For this review, take the finished solid that the model builds, in its own axes (mm). Face numbers are marked on the shaded views. A direction names the side the tool comes from. Round coordinates to 2 decimals unless told otherwise and drop trailing zeros. Loops run counter-clockwise (first coordinate to the right, second up) from the corner with the lowest first, then second, coordinate; pieces in that order, holes last. Notation, with made-up numbers: (3.25, 12.5) -> (34.25, 12.5) arc R14 ccw to (34.25, 21.5) -> close; hole circle Ø8 at (29, 75.5). An arc over 180 degrees is marked (long way). Write each question's results on one line, items separated by ' | '.
```python
from build123d import *

# Parameters (mm, degrees)
BOSS_EXTRUDE1_DEPTH = 5
SKETCH2_W           = 9
SKETCH2_H           = 5
SKETCH2_W_2         = 18
BOSS_EXTRUDE2_DEPTH = 9
SKETCH3_W           = 1.5
SKETCH3_H           = 9
SKETCH3_W_2         = 3.027864045
SKETCH3_W_3         = 2
SKETCH3_W_4         = 5.05572809
CUT_EXTRUDE1_DEPTH  = 228
BOSS_EXTRUDE3_DEPTH = 20
SKETCH5_W           = 11.583853266
SKETCH5_H           = 8
CUT_EXTRUDE3_DEPTH  = 20
SKETCH6_R           = 1.5
CUT_EXTRUDE5_DEPTH  = 25


with BuildPart() as part:
    # Sketch1 → Boss-Extrude1 (new body)
    with BuildSketch(Plane(origin=(0, 0, 0), x_dir=(1, 0, 0), z_dir=(0, 1, 0))):
        with BuildLine():
            Line((-64, 250), (-64, 0))
            ThreePointArc((-64, 0), (0, -64), (64, 0))
            Line((64, 0), (64, 250))
            ThreePointArc((64, 250), (0, 314), (-64, 250))
        make_face()
    extrude(amount=BOSS_EXTRUDE1_DEPTH)

    # Sketch2 → Boss-Extrude2 (add)
    with BuildSketch(Plane(origin=(0, 5, 0), x_dir=(1, 0, 0), z_dir=(0, 1, 0))):
        with Locations((4.5, 27.5)):
            Rectangle(SKETCH2_W, SKETCH2_H)
        with Locations((-4.5, 27.5)):
            Rectangle(SKETCH2_W, SKETCH2_H)
        with Locations((-53.5, 27.5)):
            Rectangle(SKETCH2_W, SKETCH2_H)
        with Locations((53.5, 27.5)):
            Rectangle(SKETCH2_W, SKETCH2_H)
        with Locations((53.5, 82.5)):
            Rectangle(SKETCH2_W, SKETCH2_H)
        with Locations((4.5, 82.5)):
            Rectangle(SKETCH2_W, SKETCH2_H)
        with Locations((-4.5, 82.5)):
            Rectangle(SKETCH2_W, SKETCH2_H)
        with Locations((-53.5, 82.5)):
            Rectangle(SKETCH2_W, SKETCH2_H)
        with Locations((-53.5, 137.5)):
            Rectangle(SKETCH2_W, SKETCH2_H)
        with Locations((-4.5, 137.5)):
            Rectangle(SKETCH2_W, SKETCH2_H)
        with Locations((4.5, 137.5)):
            Rectangle(SKETCH2_W, SKETCH2_H)
        with Locations((53.5, 137.5)):
            Rectangle(SKETCH2_W, SKETCH2_H)
        with Locations((53.5, 192.5)):
            Rectangle(SKETCH2_W, SKETCH2_H)
        with Locations((-53.5, 192.5)):
            Rectangle(SKETCH2_W, SKETCH2_H)
        with Locations((-53.5, 247.5)):
            Rectangle(SKETCH2_W, SKETCH2_H)
        with Locations((-4.5, 247.5)):
            Rectangle(SKETCH2_W, SKETCH2_H)
        with Locations((4.5, 247.5)):
            Rectangle(SKETCH2_W, SKETCH2_H)
        with Locations((53.5, 247.5)):
            Rectangle(SKETCH2_W, SKETCH2_H)
        with Locations((0, 192.5)):
            Rectangle(SKETCH2_W_2, SKETCH2_H)
    extrude(amount=BOSS_EXTRUDE2_DEPTH)

    # Sketch3 → Cut-Extrude1 (cut)
    with BuildSketch(Plane.XY.offset(-25)):
        with BuildLine():
            ThreePointArc((-56.5, 14), (-54.263932023, 12), (-52.027864045, 14))
            Line((-52.027864045, 14), (-56.5, 14))
        make_face()
        with Locations((-57.25, 9.5)):
            Rectangle(SKETCH3_W, SKETCH3_H)
        with Locations((-50.513932023, 9.5)):
            Rectangle(SKETCH3_W_2, SKETCH3_H)
        with Locations((-8, 9.5)):
            Rectangle(SKETCH3_W_3, SKETCH3_H)
        with BuildLine():
            Line((-2.527864045, 14), (-7, 14))
            ThreePointArc((-7, 14), (-4.763932023, 12), (-2.527864045, 14))
        make_face()
        with Locations((0, 9.5)):
            Rectangle(SKETCH3_W_4, SKETCH3_H)
        with BuildLine():
            Line((7, 14), (2.527864045, 14))
            ThreePointArc((2.527864045, 14), (4.763932023, 12), (7, 14))
        make_face()
        with Locations((8, 9.5)):
            Rectangle(SKETCH3_W_3, SKETCH3_H)
        with Locations((50.513932023, 9.5)):
            Rectangle(SKETCH3_W_2, SKETCH3_H)
        with BuildLine():
            Line((56.5, 14), (52.027864045, 14))
            ThreePointArc((52.027864045, 14), (54.263932023, 12), (56.5, 14))
        make_face()
        with Locations((57.25, 9.5)):
            Rectangle(SKETCH3_W, SKETCH3_H)
    extrude(amount=-CUT_EXTRUDE1_DEPTH, mode=Mode.SUBTRACT)

    # Sketch4 → Boss-Extrude3 (add)
    with BuildSketch(Plane.XZ):
        with BuildLine():
            Line((-64, 0), (-64, -250))
            ThreePointArc((-64, -250), (0, -314), (64, -250))
            Line((64, -250), (64, 0))
            ThreePointArc((64, 0), (0, 64), (-64, 0))
        make_face()
        with BuildLine():
            Line((-59, 0), (-59, -250))
            ThreePointArc((-59, -250), (0, -309), (59, -250))
            Line((59, -250), (59, 0))
            ThreePointArc((59, 0), (0, 59), (-59, 0))
        make_face(mode=Mode.SUBTRACT)
    extrude(amount=BOSS_EXTRUDE3_DEPTH)

    # Sketch5 → Cut-Extrude3 (cut)
    with BuildSketch(Plane(origin=(0, 5, 0), x_dir=(1, 0, 0), z_dir=(0, 1, 0))):
        with Locations((-50.708073367, 254)):
            Rectangle(SKETCH5_W, SKETCH5_H)
        with Locations((-50.708073367, 199)):
            Rectangle(SKETCH5_W, SKETCH5_H)
        with Locations((-50.708073367, 144)):
            Rectangle(SKETCH5_W, SKETCH5_H)
        with Locations((-50.708073367, 89)):
            Rectangle(SKETCH5_W, SKETCH5_H)
        with Locations((-50.708073367, 34)):
            Rectangle(SKETCH5_W, SKETCH5_H)
        with Locations((50.708073367, 144)):
            Rectangle(SKETCH5_W, SKETCH5_H)
        with Locations((50.708073367, 199)):
            Rectangle(SKETCH5_W, SKETCH5_H)
        with Locations((50.708073367, 254)):
            Rectangle(SKETCH5_W, SKETCH5_H)
        with Locations((50.708073367, 89)):
            Rectangle(SKETCH5_W, SKETCH5_H)
        with Locations((50.708073367, 34)):
            Rectangle(SKETCH5_W, SKETCH5_H)
    extrude(amount=-CUT_EXTRUDE3_DEPTH, mode=Mode.SUBTRACT)

    # Sketch6 → Cut-Extrude5 (cut)
    with BuildSketch(Plane.XZ):
        with Locations(Location((0, 54.47166112, 0), (0, 0, 270))):
            Circle(SKETCH6_R)
        with Locations(Location((0, -304.513619398, 0), (0, 0, 270))):
            Circle(SKETCH6_R)
    extrude(amount=-CUT_EXTRUDE5_DEPTH, mode=Mode.SUBTRACT)


solid = part.part
```
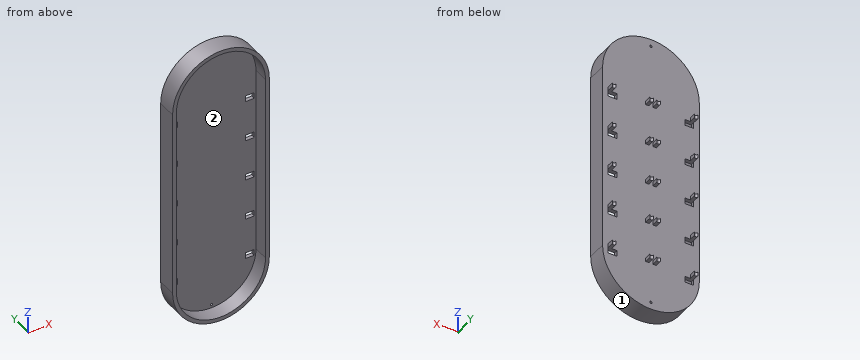
1. For pin 1 (5 mm diameter, centred on x = -5, y = 9.5, fed in from +Z); pin 2 (5.5 mm diameter, centred on y = 8.5, z = -26.5, fed in from +X); pin 3 (1.5 mm diameter, centred on y = 8.5, z = -136.5, fed in from -X), all flat-tipped, find the tip position at first contact; note any pin that passes through.
Values found:
pin 1: stops at z = -25 | pin 2: stops at x = 56.5 | pin 3: stops at x = -56.5
2. Consider section C-C (x = 29). State the section outline as (y, z) points.
Values found:
outline: (-20, -307.05) -> (5, -307.05) -> (5, 57.05) -> (-20, 57.05) -> (-20, 51.38) -> (0, 51.38) -> (0, -301.38) -> (-20, -301.38) -> close
3. Consider section B-B (z = -21.5). State the section outline as (x, y) points.
Values found:
outline: (-64, -20) -> (-59, -20) -> (-59, 0) -> (59, 0) -> (59, -20) -> (64, -20) -> (64, 5) -> (-64, 5) -> close
4. To check wall thickness, follow probe 1 along X at (y, z) = (-15, -12.5); probe 2 along Y at (x, z) = (49, -23); probe 3 along Z at (x, y) = (-52, 1). State the ranges of each line that lie inside material, in increasing order.
Values found:
probe 1: x = -64 to -59, 59 to 64 | probe 2: y = 0 to 5 | probe 3: z = -287.31 to -258, -250 to -203, -195 to -148, -140 to -93, -85 to -38, -30 to 37.31
5. Tool access review of the marked faces 1 and 2: name each direction out of +Z, -Z, +X, -X, +Y, -Y from which nothing blocks a thin tool from reaching the whole face with its end or side.
Values found:
face 1: -Z, +Y, -Y | face 2: -Y
6. Consider section A-A (y = -14.5). State the section outline as (x, z) points, plus the area to 3 significant figures.
Values found:
outline: (-64, -250) arc R64 ccw to (64, -250) -> (64, 0) arc R64 ccw to (-64, 0) -> close; hole (-59, -250) arc R59 ccw to (59, -250) -> (59, 0) arc R59 ccw to (-59, 0) -> close | area: 4,430 mm2
